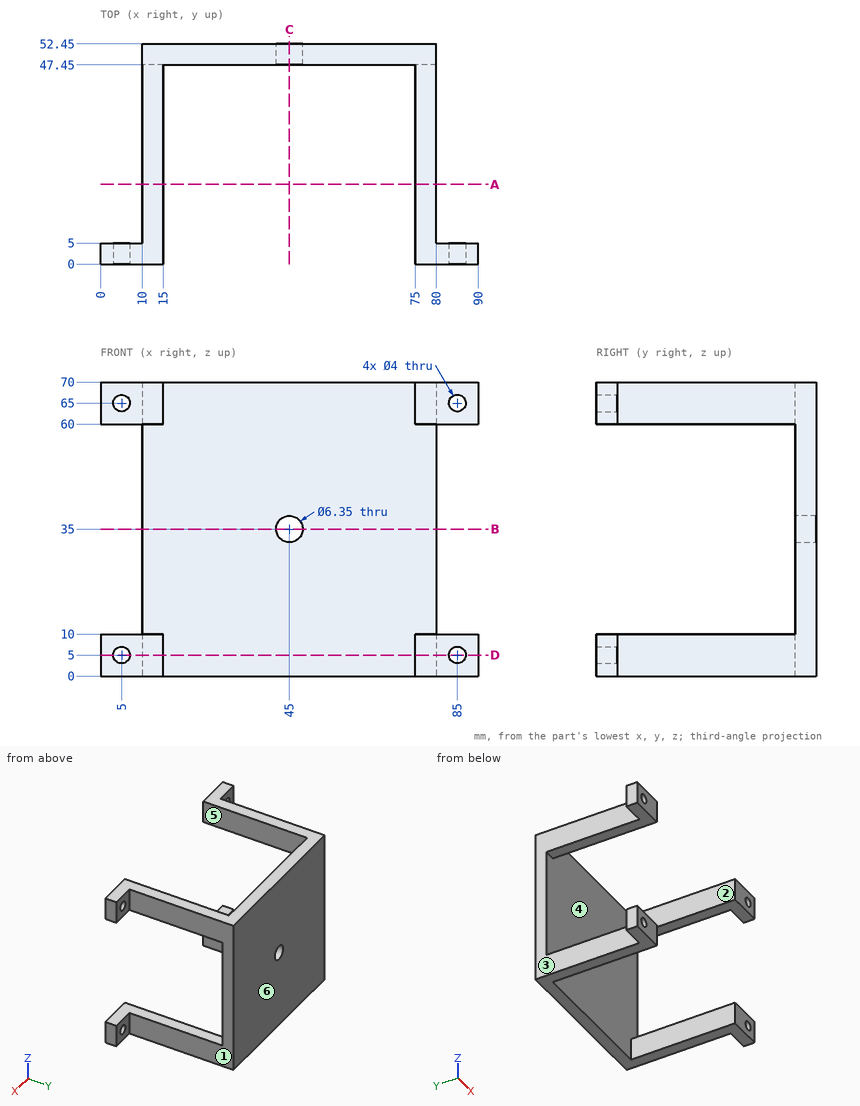
Drawing for the job (mm, zero at the part's lowest x, y, z). A direction names the side the tool comes from. Give positions to 0.01 mm unless a question says otherwise; leave off trailing zeros. Loops run counter-clockwise (first coordinate to the right, second up) from the corner with the lowest first, then second, coordinate; pieces in that order, holes last.
Item 1: Drill centre lines: line 1 along Z through (x, y) = (85, 2.6); line 2 along X through (y, z) = (3, 5); line 3 along X through (y, z) = (48.85, 35) (3 decimals). Where is each one in solid material? Low to high.
Check values:
line 1: z = 0 to 3, 7 to 10, 60 to 63, 67 to 70
line 2: x = 0 to 3, 7 to 15, 75 to 83, 87 to 90
line 3: x = 10 to 41.825, 48.175 to 80
Item 2: Which spindle directions (+Z, -Z, +X, -X, +Y, -Y) get a long thin tool onto all of the face, cutting with end or side? Do the marked faces 1 and 2. Say none if no direction does.
Check values:
face 1: +Z, -Z, +X, +Y
face 2: +Z, -Z, -Y
Item 3: Mould opens along X. For the marked faces 3, 4, 5 and 6 say: +X half, -X half, draft (parallel to the pull), parting line (faces both ways), or undercut.
Check values:
face 3: -X half
face 4: undercut
face 5: undercut
face 6: draft
Item 4: Slice it at C-C (x = 45). Write the cut outline in (y, z) (3 decimals), plus the area to 3 significant figures.
Check values:
outline: (47.45, 0) - (52.45, 0) - (52.45, 31.825) - (47.45, 31.825) - close; (47.45, 38.175) - (52.45, 38.175) - (52.45, 70) - (47.45, 70) - close
area: 318 mm2
Item 5: Slice it at A-A (y = 19). Write the cut outline in (x, z).
Check values:
outline: (10, 0) - (15, 0) - (15, 10) - (10, 10) - close; (10, 60) - (15, 60) - (15, 70) - (10, 70) - close; (75, 0) - (80, 0) - (80, 10) - (75, 10) - close; (75, 60) - (80, 60) - (80, 70) - (75, 70) - close
Item 6: Slice it at D-D (z = 5). Write the cut outline in (x, y).
Check values:
outline: (0, 0) - (3, 0) - (3, 5) - (0, 5) - close; (7, 0) - (15, 0) - (15, 47.45) - (75, 47.45) - (75, 0) - (83, 0) - (83, 5) - (80, 5) - (80, 52.45) - (10, 52.45) - (10, 5) - (7, 5) - close; (87, 0) - (90, 0) - (90, 5) - (87, 5) - close
Item 7: Slice it at B-B (z = 35). Write the cut outline in (x, y) (3 decimals), plus the area to 3 significant figures.
Check values:
outline: (10, 47.45) - (41.825, 47.45) - (41.825, 52.45) - (10, 52.45) - close; (48.175, 47.45) - (80, 47.45) - (80, 52.45) - (48.175, 52.45) - close
area: 318 mm2
Item 8: Drop flat-ended pins along their axis: P1, Ø5, axis at x = 6.5, z = 65, coming from the +Y side; P2, Ø3, axis at y = 29.5, z = 2.5, coming from the -X side; P3, Ø6, axis at y = 40, z = 12, coming from the +X side; P4, Ø12, axis at x = 83.5, y = 16, coming from the +Z side. Give the stop position or say it passes through.
Check values:
P1: stops at y = 5
P2: stops at x = 10
P3: stops at x = 80
P4: stops at z = 70
